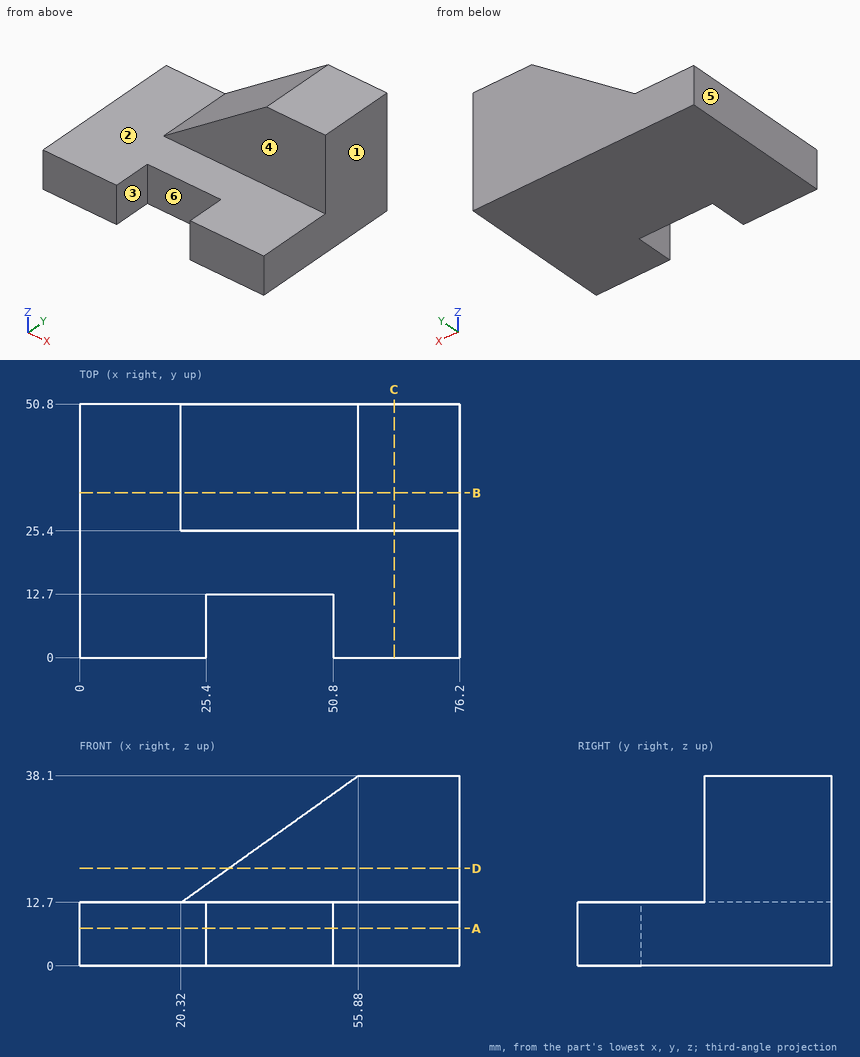
Here's the drawing with two shaded views (mm, measured from the low corner). I have some questions. A direction names the side the tool comes from. Coordinates: 2 decimals unless noted, no trailing zeros. Write each loop counter-clockwise with the first axis right and the second up, starting at its lowest first coordinate (ties: lowest second). Pieces come first, ordered by that corner, then holes. Notation, with made-up numbers: (51.25, 5.5) - (83.25, 5.5) arc R10 cw to (83.25, 15.5) - close; hole circle Ø10 at (37, 57). An arc over 180 degrees is marked (long way). Return JSON: item names as keys, results as strings.
Q1. If we section it at B-B (y = 33): Please give me the cut outline in (x, z), then the cut area to 3 significant figures.
Computed values:
{"outline": "(0, 0) - (76.2, 0) - (76.2, 38.1) - (55.88, 38.1) - (20.32, 12.7) - (0, 12.7) - close", "area": "1,940 mm2"}
Q2. On a 3-axis mill with a long thin cutter (end or side, diameter ignored), from which of +Z, -Z, +X, -X, +Y, -Y can I reach the whole of each face in a straight line? I mean the marked faces 1, 2 and 3. Say none if no direction works.
Computed values:
{"face 1": "+Z, -Z, +X, +Y, -Y", "face 2": "+Z, -X, -Y", "face 3": "+Z, -Z, -Y"}
Q3. If we section it at A-A (z = 7.5): Please give me the cut outline in (x, y).
Computed values:
{"outline": "(0, 0) - (25.4, 0) - (25.4, 12.7) - (50.8, 12.7) - (50.8, 0) - (76.2, 0) - (76.2, 50.8) - (0, 50.8) - close"}
Q4. If we section it at D-D (z = 19.5): Please give me the cut outline in (x, y), then the cut area to 3 significant figures.
Computed values:
{"outline": "(29.84, 25.4) - (76.2, 25.4) - (76.2, 50.8) - (29.84, 50.8) - close", "area": "1,180 mm2"}
Q5. Please list where these lines run through material, in increasing order: L1, parallel to Y at x = 42, z = 27.5; L2, parallel to Z at x = 28.5, y = 17.5; L3, parallel to Y at x = 34, z = 4. Write a range as from..to.
Computed values:
{"L1": "y = 25.4..50.8", "L2": "z = 0..12.7", "L3": "y = 12.7..50.8"}
Q6. I'm going to push flat-ended pins straight in: pin 1 Ø10 at (x, z) = (64, 10) entering from -Y; pin 2 Ø1.5 at (y, z) = (40, 16) entering from -X; pin 3 Ø4 at (x, z) = (43.5, 4) entering from -Y; pin 4 Ø7.5 at (x, z) = (57.5, 21) entering from -Y. Where does each tip first touch, or does it pass through?
Computed values:
{"pin 1": "stops at y = 0", "pin 2": "stops at x = 23.89", "pin 3": "stops at y = 12.7", "pin 4": "stops at y = 25.4"}
Q7. Thinking about a two-plate mould opening in X: for the marked faces 4, 5 and 6, which applies, +X half, -X half, draft (parallel to the pull), parting line (faces both ways), or undercut?
Computed values:
{"face 4": "draft", "face 5": "-X half", "face 6": "undercut"}
Q8. If we section it at C-C (x = 63): Please give me the cut outline in (y, z), then the cut area to 3 significant figures.
Computed values:
{"outline": "(0, 0) - (50.8, 0) - (50.8, 38.1) - (25.4, 38.1) - (25.4, 12.7) - (0, 12.7) - close", "area": "1,290 mm2"}
